Autodesk Inventor part; units mm, degrees
ref_plane "Work Plane1" through (0, 0, 150) normal (0, 0, 1) x (1, 0, 0)
ref_plane "Work Plane2" through (0, 0, 80) normal (0, 0, 1) x (1, 0, 0)
ref_plane "YZ Plane" through (0, 0, 0) normal (1, 0, 0) x (0, 1, 0)
sketch "Sketch1" plane through (0, 0, 0) normal (0, 0, 1) x (1, 0, 0)
  circle A0 centre (0, 0) radius 30
  dimension "d0" = 60
extrude "Extrusion1" add sketch "Sketch1" along normal blind 160
ref_plane "Work Plane1" through (0, 0, 150) normal (0, 0, 1) x (1, 0, 0)
sketch "Sketch4" plane through (0, 0, 150) normal (0, 0, 1) x (1, 0, 0)
  circle A0 centre (0, 0) radius 30
  line L0 (0, 0) -> (21.5, 37.2391)
  line L1 (0, 0) -> (43, 0) construction
  line L2 (0, 0) -> (-25, 43.3013)
  arc A1 (21.5, 37.2391) -> (-21.5, 37.2391) centre (0, 0) ccw
  point P0 (-21.5, 37.2391)
  point P1 (-15, 25.9808)
  point P2 (15, 25.9808)
  dimension "d6" = 43
  dimension "d7" = 60
extrude "Extrusion2" add sketch "Sketch4" against normal blind 30 contours A0 L2 A1 L0
ref_plane "Work Plane2" through (0, 0, 80) normal (0, 0, 1) x (1, 0, 0)
mirror "Mirror1" about plane through (0, 0, 80) normal (0, 0, 1) of "Extrusion2"
sketch "Sketch5" plane through (0, 0, 80) normal (0, 0, 1) x (1, 0, 0)
  line L0 (0, 0) -> (21.5, -37.2391)
  line L1 (0, 0) -> (43, 0) construction
  circle A0 centre (0, 0) radius 30
  line L2 (0, 0) -> (-21.5, -37.2391)
  arc A1 (-21.5, -37.2391) -> (21.5, -37.2391) centre (0, 0) ccw
  point P0 (15, -25.9808)
  point P1 (-15, -25.9808)
  dimension "d10" = 43
  dimension "d11" = 60
extrude "Extrusion3" add sketch "Sketch5" along normal mid plane 40 contours L0 A1 L2 A0
chamfer "Chamfer1" distance 5 angle 45 6 edges at (0, 43, 150) (0, 43, 120) (0, 43, 40) (0, 43, 10) (0, -43, 100) (0, -43, 60)
chamfer "Chamfer2" distance 2 angle 45 2 edges at (-30, 0, 0) (-30, 0, 160)
sketch "Sketch6" plane through (0, 0, 160) normal (0, 0, 1) x (1, 0, 0)
  circle A0 centre (0, 0) radius 10
  dimension "d20" = 20
extrude "Extrusion4" add sketch "Sketch6" along normal blind 40 and the other way blind 200
Work out the finished part from the listing and answer in its coordinate system (mm). A direction names the side the tool comes from. Round coordinates to 2 decimals unless told otherwise and drop trailing zeros. Write each loop counter-clockwise with the first axis right and the second up, starting at its lowest first coordinate (ties: lowest second). Pieces come first, ordered by that corner, then holes.
1) A cutting plane is placed at B-B on y = 0. Determine the outline of the cut face in (x, z), and give its area (3 significant figures).
2) Flat-ended cylindrical pins translate along their axes: P1, Ø5, axis at y = -22.5, z = 20.5, coming from the +X side; P2, Ø1.5, axis at y = -5.5, z = 118, coming from the -X side; P3, Ø10, axis at x = 6, y = 20.5, coming from the +Z side. Find the tip coordinate at first contact, or state that the pin passes through.
3) Consider probe 1 along Y at (x, z) = (1, 186.5); probe 2 along Z at (x, y) = (-17.5, 14); probe 3 along Y at (x, z) = (1.5, 28). Determine where each line is inside the solid, lowest interval first.
4) Which of the six approach directions +Z, -Z, +X, -X, +Y, -Y give full straight-line access (tool end or side, diameter ignored) to faces 5 (the face through (0, -12, 160)), 6 (the face through (0, -12, 0)), 7 (the face through (-18.3, 31.7, 24.8)), 8 (the face through (18.204, -31.531, 79.72))?
5) Determine the mould class of faces 1 (the face through (0, 33, 120)), 2 (the face through (0, -39, 99)), 3 (the face through (-18.204, 31.531, 135.21)), 4 (the face through (-6.1, -27.46, 0.13)) for opening direction Y: pulls with the +Y half, pulls with the -Y half, needs draft (parallel to the pull), parting line crosses it, or undercut.
6) A cutting plane is placed at C-C on z = 92.5. Determine the outline of the cut face in (x, y), and give its area (3 significant figures).
Entries:
1. outline: (-30, 2) - (-28, 0) - (-10, 0) - (-10, -40) - (10, -40) - (10, 0) - (28, 0) - (30, 2) - (30, 158) - (28, 160) - (10, 160) - (10, 200) - (-10, 200) - (-10, 160) - (-28, 160) - (-30, 158) - close
1. area: 11,200 mm2
2. P1: stops at x = 22.36
2. P2: stops at x = -29.62
2. P3: stops at z = 160
3. probe 1: y = -9.95 to 9.95
3. probe 2: z = 0 to 160
3. probe 3: y = -29.96 to 42.97
4. face 5: +Z
4. face 6: -Z
4. face 7: +Z, -Z, -X
4. face 8: +Z, -Z, +X
5. face 1: needs draft
5. face 2: pulls with the -Y half
5. face 3: undercut
5. face 4: parting line crosses it
6. outline: (-21.5, -37.24) arc R43 ccw to (21.5, -37.24) - (15, -25.98) arc R30 ccw (long way) to (-15, -25.98) - close
6. area: 3,320 mm2
